CAD build for the part. Positions are in the model's coordinates, mm. A direction names the side the tool comes from. Give positions to 0.01 mm unless a question says otherwise; leave off trailing zeros. Write each loop counter-clockwise with the first axis right and the second up, starting at its lowest first coordinate (ties: lowest second). Pieces come first, ordered by that corner, then holes. Notation, with made-up numbers: (-33.75, -33.75) -> (-0.75, -33.75) arc R13 ccw to (-0.75, -9.75) -> close; hole circle Ø3 at (-32.75, 38). An arc over 180 degrees is marked (long way). Answer as a JSON object with one key per item and string values.
```python
from build123d import *

# Parameters (mm, degrees)
BOSS_EXTRU_5_DEPTH      = 10
ESQUISSE1_W             = 36
ESQUISSE1_H             = 20
ESQUISSE1_W_2           = 2
BOSS_EXTRU_6_DEPTH      = 12
ESQUISSE1_9_W           = 36
ESQUISSE1_9_H           = 20
ENL_V_MAT_EXTRU_4_DEPTH = 10
ESQUISSE1_10_R          = 1.7
ENL_V_MAT_EXTRU_5_DEPTH = 55.295487842


with BuildPart() as part:
    # Esquisse3 → Boss.-Extru.5 (new, symmetric)
    with BuildSketch(Plane.XY):
        Polygon((-36, 0), (-52, -2.958401047), (-52, -0.992722896), (-36, 2), align=None)
    boss_extru_5 = extrude(amount=BOSS_EXTRU_5_DEPTH, both=True)

    # Esquisse1 → Boss.-Extru.6 (add)
    with BuildSketch(Plane(origin=(0, 0, 0), x_dir=(1, 0, 0), z_dir=(0, 1, 0))):
        with Locations((-18, 0)):
            Rectangle(ESQUISSE1_W, ESQUISSE1_H)
        with Locations((-37, 0)):
            Rectangle(ESQUISSE1_W_2, ESQUISSE1_H)
    boss_extru_6 = extrude(amount=BOSS_EXTRU_6_DEPTH)

    # Esquisse1_9 → Enl_v. mat.-Extru.4 (cut)
    with BuildSketch(Plane(origin=(0, 0, 0), x_dir=(1, 0, 0), z_dir=(0, 1, 0))):
        with Locations((-18, 0)):
            Rectangle(ESQUISSE1_9_W, ESQUISSE1_9_H)
    enl_v_mat_extru_4 = extrude(amount=ENL_V_MAT_EXTRU_4_DEPTH, mode=Mode.SUBTRACT)

    # Esquisse1_10 → Enl_v. mat.-Extru.5 (cut, symmetric)
    with BuildSketch(Plane(origin=(0, 0, 0), x_dir=(1, 0, 0), z_dir=(0, 1, 0))):
        with Locations((-47, 0)):
            Circle(ESQUISSE1_10_R)
    enl_v_mat_extru_5 = extrude(amount=ENL_V_MAT_EXTRU_5_DEPTH, both=True, mode=Mode.SUBTRACT)

    # Sym_trie4: Boss.-Extru.5, Boss.-Extru.6, Enl_v. mat.-Extru.4, Enl_v. mat.-Extru.5 across plane
    add(boss_extru_5.mirror(Plane(origin=(0, 0, 0), x_dir=(0, 0, 1), z_dir=(1, 0, 0))))
    add(boss_extru_6.mirror(Plane(origin=(0, 0, 0), x_dir=(0, 0, 1), z_dir=(1, 0, 0))))
    add(enl_v_mat_extru_4.mirror(Plane(origin=(0, 0, 0), x_dir=(0, 0, 1), z_dir=(1, 0, 0))), mode=Mode.SUBTRACT)
    add(enl_v_mat_extru_5.mirror(Plane(origin=(0, 0, 0), x_dir=(0, 0, 1), z_dir=(1, 0, 0))), mode=Mode.SUBTRACT)


solid = part.part
```
1) 3-axis set-ups, long thin cutter, end or side, ignore diameter. For faces 4 (the flat face through (36, 5, 0)), 5 (the flat face through (-38, 7, 0)), 6 (the cylindrical face through (-48.7, -1.04, -0.07)), 7 (the flat face through (38, 7, 0)), 8 (the flat face through (-52, -2, 0)): which of +Z, -Z, +X, -X, +Y, -Y reach the whole face in a straight line?
Model answer:
{"face 4": "+Z, -Z, -Y", "face 5": "+Z, -Z, -X, +Y", "face 6": "+Y, -Y", "face 7": "+Z, -Z, +X, +Y", "face 8": "+Z, -Z, -X, +Y, -Y"}
2) Slice it at D-D (z = 7.5). List the corners of the cut face in (x, y), then the cut area to 3 significant figures.
Model answer:
{"outline": "(-52, -2.96) -> (-36, 0) -> (-36, 10) -> (36, 10) -> (36, 0) -> (52, -2.96) -> (52, -0.99) -> (38, 1.63) -> (38, 12) -> (-38, 12) -> (-38, 1.63) -> (-52, -0.99) -> close", "area": "248 mm2"}
3) Mould opens along X. For faces 1 (the cylindrical face through (48.7, -1.04, -0.07)), 2 (the flat face through (-45.098, 0.298, 0.14)), 3 (the flat face through (1, 12, 0)) say: released by +X, released by -X, zero draft, split by the parting line, or undercut.
Model answer:
{"face 1": "undercut", "face 2": "released by -X", "face 3": "zero draft"}
4) Slice it at A-A (y = 2.5). List the corners of the cut face in (x, z).
Model answer:
{"outline": "(-38, -10) -> (-36, -10) -> (-36, 10) -> (-38, 10) -> close; (36, -10) -> (38, -10) -> (38, 10) -> (36, 10) -> close"}
5) Slice it at C-C (x = -47). List the corners of the cut face in (y, z).
Model answer:
{"outline": "(-2.03, -10) -> (-0.06, -10) -> (-0.06, -1.7) -> (-2.03, -1.7) -> close; (-2.03, 1.7) -> (-0.06, 1.7) -> (-0.06, 10) -> (-2.03, 10) -> close"}
6) Wall check: probe 1 along Z at (x, y) = (47, -0.75); probe 2 along X at (y, z) = (6, 6.75); probe 3 along Y at (x, z) = (6, -6.5). Give the ranges that are in metal, low to high.
Model answer:
{"probe 1": "z = -10 to -1.7, 1.7 to 10", "probe 2": "x = -38 to -36, 36 to 38", "probe 3": "y = 10 to 12"}
7) Pin check, flat tips, straight feed: pin 1 (1.5 mm diameter, centred on y = 4.5, z = 6.5, fed in from +X); pin 2 (2 mm diameter, centred on x = 47, z = 0, fed in from -Y); pin 3 (8 mm diameter, centred on y = 6.5, z = -0.5, fed in from -X); pin 4 (6 mm diameter, centred on x = -2.5, z = -1.5, fed in from -Y). Stop position of each tip, or through.
Model answer:
{"pin 1": "stops at x = 38", "pin 2": "passes through", "pin 3": "stops at x = -38", "pin 4": "stops at y = 10"}
8) Slice it at B-B (z = 0). List the corners of the cut face in (x, y), then the cut area to 3 significant figures.
Model answer:
{"outline": "(-52, -2.96) -> (-48.7, -2.35) -> (-48.7, -0.38) -> (-52, -0.99) -> close; (-45.3, -1.72) -> (-36, 0) -> (-36, 10) -> (36, 10) -> (36, 0) -> (45.3, -1.72) -> (45.3, 0.26) -> (38, 1.63) -> (38, 12) -> (-38, 12) -> (-38, 1.63) -> (-45.3, 0.26) -> close; (48.7, -2.35) -> (52, -2.96) -> (52, -0.99) -> (48.7, -0.38) -> close", "area": "235 mm2"}
